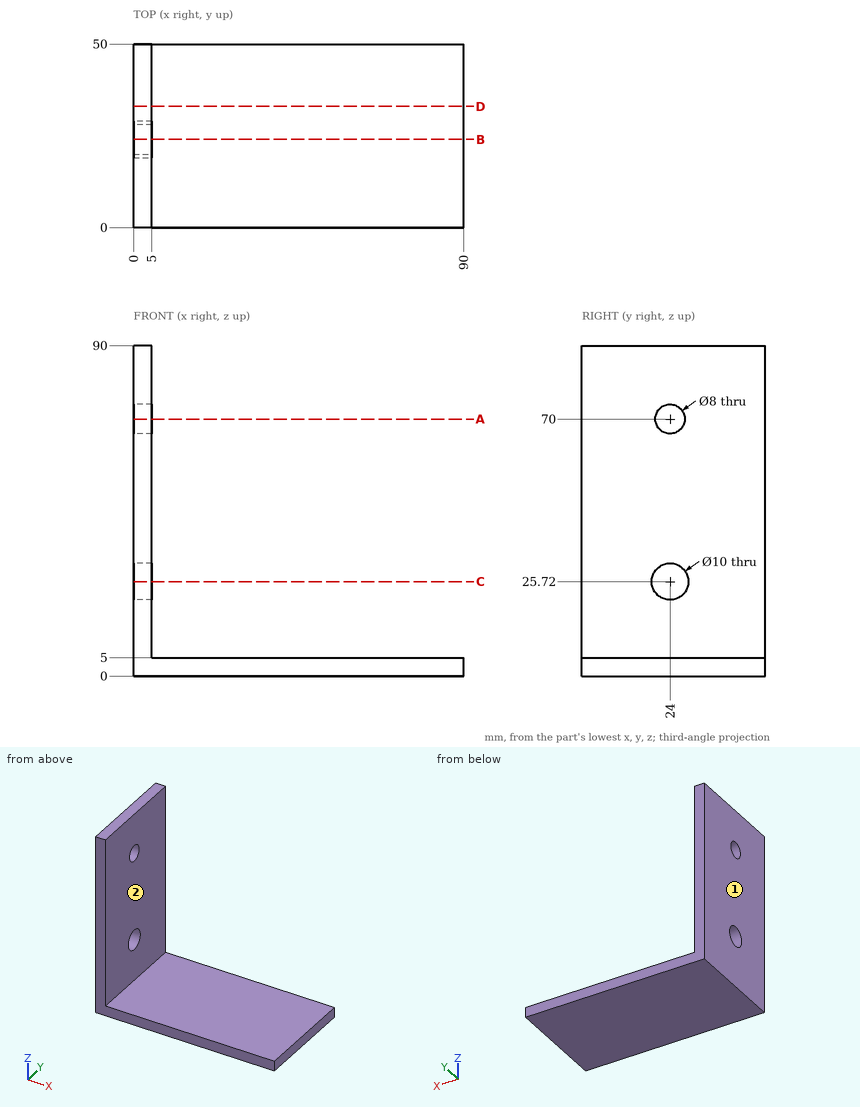
Here's the drawing with two shaded views (mm, measured from the low corner). I have some questions. A direction names the side the tool comes from. Coordinates: 2 decimals unless noted, no trailing zeros. Loops run counter-clockwise (first coordinate to the right, second up) from the corner with the lowest first, then second, coordinate; pieces in that order, holes last. Notation, with made-up numbers: (-6, 75.25) - (47, 75.25) arc R26 cw to (47, 109.25) - close; hole circle Ø7 at (6, 33.5). An arc over 180 degrees is marked (long way). Answer as CSV lines item,"result". Start each with the question number.
1) Suppose I cut it at B-B (y = 24). Please give me the cut outline in (x, z).
2) Which directions (+Z, -Z, +X, -X, +Y, -Y) give clear straight access to the entire face, cutting with the end or side of a thin tool? Please do the marked faces 1 and 2.
3) Suppose I cut it at C-C (z = 25.72). Please give me the cut outline in (x, y), plus the area to 3 significant figures.
4) For pin 1 (5 mm diameter, centred on x = 65.5, y = 44.5, fed in from +Z); pin 2 (1 mm diameter, centred on y = 5.5, z = 63.5, fed in from +X), each with a flat end and sliding along its axis, tell me the tip position at first contact or that it passes through.
5) Suppose I cut it at D-D (y = 33). Please give me the cut outline in (x, z).
6) Suppose I cut it at A-A (z = 70). Please give me the cut outline in (x, y).
7) I need wall thicknesses on line 1 (Z direction, x = 3.5, y = 24); line 2 (X direction, y = 24.5, z = 45); line 3 (Y direction, x = 2, z = 25). Which ranges of each line are inside material? Lowest first, please. Write a range as from..to.
Check result:
1,outline,"(0, 0) - (90, 0) - (90, 5) - (5, 5) - (5, 20.72) - (0, 20.72) - close; (0, 30.72) - (5, 30.72) - (5, 66) - (0, 66) - close; (0, 74) - (5, 74) - (5, 90) - (0, 90) - close"
2,face 1,"+Z, -Z, -X, +Y, -Y"
2,face 2,"+Z, +X, +Y, -Y"
3,outline,"(0, 0) - (5, 0) - (5, 19) - (0, 19) - close; (0, 29) - (5, 29) - (5, 50) - (0, 50) - close"
3,area,"200 mm²"
4,pin 1,"stops at z = 5"
4,pin 2,"stops at x = 5"
5,outline,"(0, 0) - (90, 0) - (90, 5) - (5, 5) - (5, 90) - (0, 90) - close"
6,outline,"(0, 0) - (5, 0) - (5, 20) - (0, 20) - close; (0, 28) - (5, 28) - (5, 50) - (0, 50) - close"
7,line 1,"z = 0..20.72, 30.72..66, 74..90"
7,line 2,"x = 0..5"
7,line 3,"y = 0..19.05, 28.95..50"
